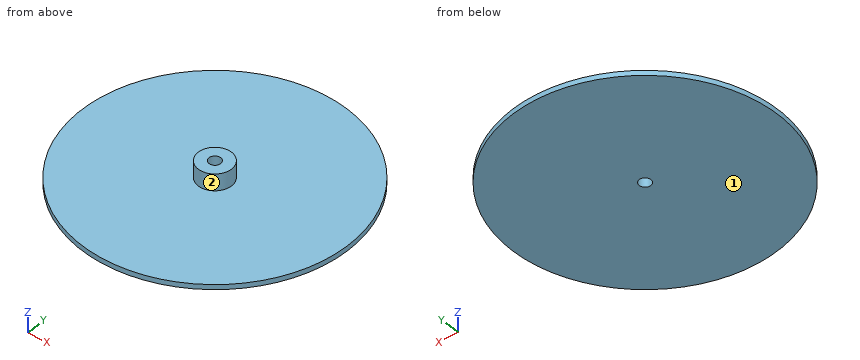
Autodesk Fusion 360 part; units mm, degrees
sketch "スケッチ1" plane through (0, 0, 0) normal (0, 0, 1) x (1, 0, 0)
  circle A0 centre (0, 0) radius 80
  circle A1 centre (0, 0) radius 3.5
  dimension "d1" = 160
  dimension "d7" = 7
extrude "押し出し1" add sketch "スケッチ1" along normal blind 3 contours A0 | A1
sketch "スケッチ2" plane through (0, 0, 3) normal (0, 0, 1) x (-1, 0, 0)
  circle A0 centre (0, 0) radius 80
  circle A1 centre (0, 0) radius 10
  dimension "d4" = 20
extrude "押し出し2" add sketch "スケッチ2" along normal blind 10 contours A1
extrude "押し出し3" cut sketch "スケッチ1" along normal blind 13 contours A1
For this review, take the finished solid that the model builds, in its own axes (mm). Face numbers are marked on the shaded views. A direction names the side the tool comes from. Give positions to 0.01 mm unless a question says otherwise; leave off trailing zeros. Write each loop counter-clockwise with the first axis right and the second up, starting at its lowest first coordinate (ties: lowest second). Pieces come first, ordered by that corner, then holes.
Item 1: Take a section at C-C (z = 5). Give the boundary of the cut face in (x, y).
Item 2: Insertion check: P1, Ø3, axis at x = 0.5, z = 5, coming from the -Y side; P2, Ø5.5, axis at x = 0, y = 0, coming from the -Z side. Each pin has a flat end and moves straight along its axis. Give the tip position at first contact, or say it passes through.
Item 3: Take a section at A-A (y = 0). Give the boundary of the cut face in (x, z), and give its area (3 significant figures).
Item 4: Take a section at D-D (y = 55). Give the boundary of the cut face in (x, z), and give its area (3 significant figures).
Item 5: Machinability: for the marked faces 1 and 2, which of the approach directions +Z, -Z, +X, -X, +Y, -Y give a long, thin tool a straight path to every point of the face, cutting with its end or side? Answer none if there is none.
Item 6: Wall thickness on probe 1 along Y at (x, z) = (0, 3.25); probe 2 along Z at (x, y) = (63, 26.5); probe 3 along X at (y, z) = (-8, 9.5): over which ranges is each line inside the solid? List them lowest first.
Established:
1. outline: circle Ø20 at (0, 0); hole circle Ø7 at (0, 0)
2. P1: stops at y = -10
2. P2: passes through
3. outline: (-80, 0) - (-3.5, 0) - (-3.5, 13) - (-10, 13) - (-10, 3) - (-80, 3) - close; (3.5, 0) - (80, 0) - (80, 3) - (10, 3) - (10, 13) - (3.5, 13) - close
3. area: 589 mm2
4. outline: (-58.09, 0) - (58.09, 0) - (58.09, 3) - (-58.09, 3) - close
4. area: 349 mm2
5. face 1: -Z, +X, -X, +Y, -Y
5. face 2: +Z
6. probe 1: y = -10 to -3.5, 3.5 to 10
6. probe 2: z = 0 to 3
6. probe 3: x = -6 to 6
